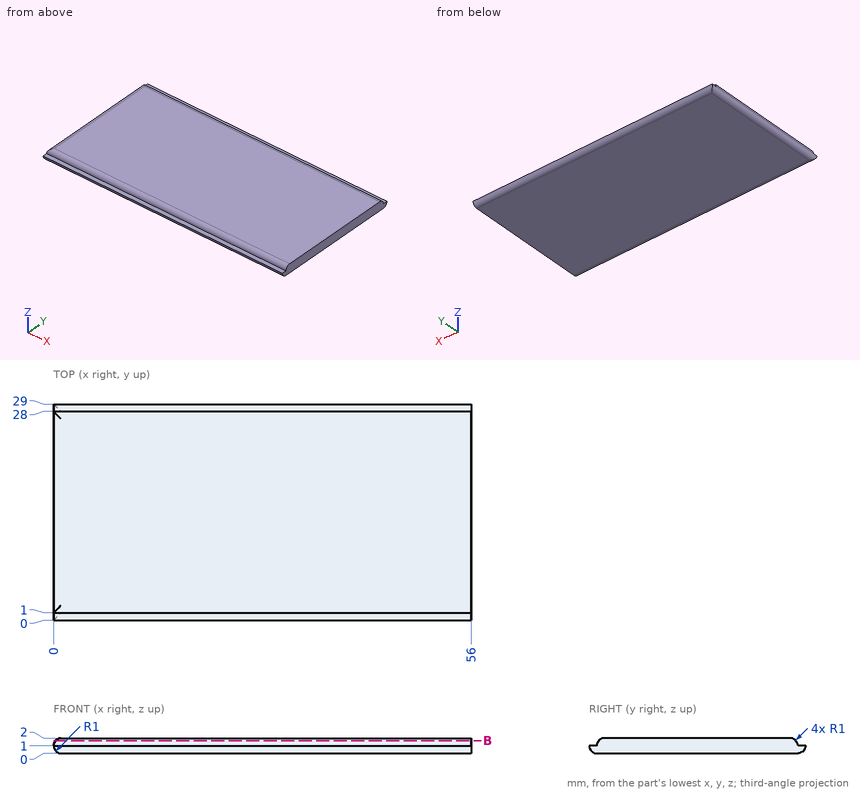
Can you work these out from the drawing? Everything is in mm from the part's minimum corner. Coordinates: 2 decimals unless noted, no trailing zeros. Order: outer loops, then holes, each group sorted by start corner. A loop starts at its lowest first (then second) coordinate and runs counter-clockwise, first axis right, second up. Notation, with made-up numbers: (58, -23) -> (77, -23) arc R21 cw to (77, -17) -> close; hole circle Ø2 at (55, 67). An arc over 180 degrees is marked (long way). Use one line per item in the form item = value.
Q1. Imagine slicing it at B-B, the plane z = 1.7. List the corners of the cut face in (x, y) for me.
From the geometry:
outline = (0.29, 1.29) -> (56, 1.29) -> (56, 27.71) -> (0.29, 27.71) -> close
Q2. Will this pin go through, and if not, where does the flat tip stop? P1, Ø0.8, axis at x = 34, y = 0.5, coming from the +Z side.
From the geometry:
P1 = 1
Q3. I need wall thicknesses on L1, parallel to X at y = 4.25, z = 0.95; L2, parallel to Y at x = 23.5, z = 0.95; L3, parallel to Y at x = 39.5, z = 1.8. Which ranges of each line are inside material? Lowest first, please.
From the geometry:
L1 = 0 to 56
L2 = 0 to 29
L3 = 1.4 to 27.6
